Could you check a few things on this model? Use its own coordinates, in mm. Face numbers are marked on the shaded views. A direction names the side the tool comes from. Coordinates: 2 decimals unless noted, no trailing zeros. Loops run counter-clockwise (first coordinate to the right, second up) from the corner with the lowest first, then second, coordinate; pieces in that order, holes last. Notation, with made-up numbers: (18, 13.5) -> (44, 13.5) arc R14 ccw to (44, 22.5) -> close; hole circle Ø3 at (-19.5, 49.5). An arc over 180 degrees is marked (long way). One line per question, with ' | ' between items. Start each with the question number.
(1) Suppose I cut it at C-C (z = 0). Please give me the cut outline in (x, y), plus the area to 4 significant figures.
(2) Suppose I cut it at D-D (x = -13). Please give me the cut outline in (y, z).
(3) If we mould it in two halves opening along Z, with no side actions, what happens to the marked faces 1, 2, 3 and 4? For each: pulls with the +Z half, pulls with the -Z half, needs draft (parallel to the pull), parting line crosses it, or undercut.
(4) Suppose I cut it at A-A (x = 0). Please give me the cut outline in (y, z), plus the area to 4 significant figures.
(5) I'm going to push flat-ended pins straight in: pin 1 Ø3.5 at (x, z) = (-13, -13) entering from -Y; pin 2 Ø10.5 at (x, z) = (1.5, -5.5) entering from +Y. Where does each tip first touch, or does it pass through?
(6) If I drill on line 1 along Z through (x, y) = (-13, -5.25); line 2 along Y through (x, z) = (2.5, -13); line 3 along X through (y, z) = (-9.25, -12), over which ranges is the centre line in solid material (lowest first)?
(7) Which directions (+Z, -Z, +X, -X, +Y, -Y) give clear straight access to the entire face, cutting with the end or side of a thin tool? Please do the marked faces 5, 6 and 7.
(8) Suppose I cut it at B-B (y = -3). Please give me the cut outline in (x, z).
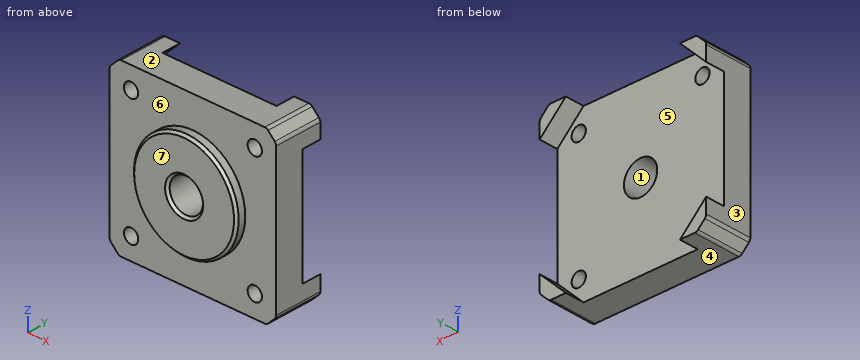
```python
from build123d import *

# Parameters (mm, degrees)
F0_W      = 35
F0_H      = 35
F1_DEPTH  = 10
F2_SIZE   = 2
F3_R      = 11
F4_DEPTH  = 0.5
F5_R      = 11
F6_DEPTH  = 2.5
F7_R      = 3.5
F8_DEPTH  = 12.001
F9_R      = 1
F10_SIZE  = 0.5
F11_R     = 1.5
F12_DEPTH = 10.001
F14_DEPTH = 4


with BuildPart() as f1:
    # F0 (on Front) → F1 (new body)
    with BuildSketch(Plane.XZ):
        Rectangle(F0_W, F0_H)
    extrude(amount=F1_DEPTH)

    # F2
    f2_edges = [f1.edges().sort_by_distance(p)[0] for p in [
        (-17.5, -5, 17.5),
        (17.5, -5, 17.5),
        (17.5, -5, -17.5),
        (-17.5, -5, -17.5),
    ]]
    chamfer(f2_edges, length=F2_SIZE)

    # F3 (on face) → F4 (cut)
    with BuildSketch(Plane.XZ.offset(10)):
        Circle(F3_R)
    extrude(amount=-F4_DEPTH, mode=Mode.SUBTRACT)

    # F5 (on face) → F6 (join)
    with BuildSketch(Plane.XZ.offset(9.5)):
        Circle(F5_R)
    extrude(amount=F6_DEPTH)

    # F7 (on face) → F8 (cut, through all)
    with BuildSketch(Plane.XZ.offset(12)):
        Circle(F7_R)
    extrude(amount=-F8_DEPTH, mode=Mode.SUBTRACT)

    # F9
    f9_edges = [f1.edges().sort_by_distance(p)[0] for p in [
        (-15.5, -5, 17.5),
        (15.5, -5, 17.5),
        (17.5, -5, 15.5),
        (17.5, -5, -15.5),
        (15.5, -5, -17.5),
        (-15.5, -5, -17.5),
        (-17.5, -5, -15.5),
        (-17.5, -5, 15.5),
    ]]
    fillet(f9_edges, radius=F9_R)

    # F10
    f10_edges = [f1.edges().sort_by_distance(p)[0] for p in [
        (-11, -12, 0),
        (-3.5, -12, 0),
    ]]
    chamfer(f10_edges, length=F10_SIZE)

    # F11 (on face) → F12 (cut, through all)
    with BuildSketch(Plane.XZ.offset(10)):
        with Locations((-13, 13)):
            Circle(F11_R)
        with Locations((-13, -13)):
            Circle(F11_R)
        with Locations((13, -13)):
            Circle(F11_R)
        with Locations((13, 13)):
            Circle(F11_R)
    extrude(amount=-F12_DEPTH, mode=Mode.SUBTRACT)

    # F13 (on face) → F14 (cut)
    with BuildSketch(Plane(origin=(0, 0, 0), x_dir=(-1, 0, 0), z_dir=(0, 1, 0))):
        Polygon((12, 17.5), (-12, 17.5), (-17.5, 12), (-17.5, -12), (-12, -17.5), (12, -17.5), (17.5, -12), (17.5, 12), align=None)
    extrude(amount=-F14_DEPTH, mode=Mode.SUBTRACT)


solid = f1.part
```
Checks:
1) outline: (-17.5, -10) -> (-11, -10) -> (-11, -11.5) -> (-10.5, -12) -> (-4, -12) -> (-3.5, -11.5) -> (-3.5, -4) -> (-17.5, -4) -> close; (3.5, -11.5) -> (4, -12) -> (10.5, -12) -> (11, -11.5) -> (11, -10) -> (17.5, -10) -> (17.5, -4) -> (3.5, -4) -> close | area: 197.5 mm^2
2) outline: (-10, -17.5) -> (0, -17.5) -> (0, -16.5) -> (-4, -16.5) -> (-4, -14.5) -> (-10, -14.5) -> close; (-10, -11.5) -> (-4, -11.5) -> (-4, 11.5) -> (-10, 11.5) -> close; (-10, 14.5) -> (-4, 14.5) -> (-4, 16.5) -> (0, 16.5) -> (0, 17.5) -> (-10, 17.5) -> close
3) face 1: undercut | face 2: pulls with the +Z half | face 3: needs draft | face 4: pulls with the -Z half
4) outline: (-12, -10.5) -> (-11.5, -11) -> (-10, -11) -> (-10, -17.5) -> (-4, -17.5) -> (-4, -3.5) -> (-11.5, -3.5) -> (-12, -4) -> close; (-12, 4) -> (-11.5, 3.5) -> (-4, 3.5) -> (-4, 17.5) -> (-10, 17.5) -> (-10, 11) -> (-11.5, 11) -> (-12, 10.5) -> close | area: 197.5 mm^2
5) pin 1: stops at y = -10 | pin 2: stops at y = -4
6) line 1: z = -17.5 to -14.5, -11.5 to 11.5, 14.5 to 17.5 | line 2: y = -10 to -4 | line 3: x = -17.5 to -14.12, -11.88 to 11.88, 14.12 to 17.5
7) face 5: +Y | face 6: -Y | face 7: +Z, -Z, +X, -X, -Y
8) outline: (-17.5, -15.09) arc R1 ccw to (-17.21, -15.79) -> (-15.79, -17.21) arc R1 ccw to (-15.09, -17.5) -> (-12, -17.5) -> (-17.5, -12) -> close; (-17.5, 12) -> (-12, 17.5) -> (-15.09, 17.5) arc R1 ccw to (-15.79, 17.21) -> (-17.21, 15.79) arc R1 ccw to (-17.5, 15.09) -> close; (12, -17.5) -> (15.09, -17.5) arc R1 ccw to (15.79, -17.21) -> (17.21, -15.79) arc R1 ccw to (17.5, -15.09) -> (17.5, -12) -> close; (12, 17.5) -> (17.5, 12) -> (17.5, 15.09) arc R1 ccw to (17.21, 15.79) -> (15.79, 17.21) arc R1 ccw to (15.09, 17.5) -> close
